Build history of the part. All positions in model axes, mm. A direction names the side the tool comes from. Give positions to 0.01 mm unless a question says otherwise; leave off trailing zeros. Order: outer loops, then holes, each group sorted by start corner. A loop starts at its lowest first (then second) coordinate and runs counter-clockwise, first axis right, second up. Notation, with made-up numbers: (86.5, 33) - (142.5, 33) arc R17 cw to (142.5, 57) - close; hole circle Ø11 at (29, 26.5). An arc over 180 degrees is marked (long way). Use a Markdown table: item, result. Add a question column.
(1) Slice it at A-A (y = 9). Write the cut outline in (x, z), then the cut area to 3 significant figures.
(2) Wall check: line 1 (X direction, y = 3, z = 0); line 2 (X direction, y = 7.75, z = 0); line 3 (Z direction, x = -2, y = 7.25). Give the ranges that are in metal, low to high.
(3) Slice it at B-B (z = 0). Write the cut outline in (x, y) (1 decimal), then the cut area to 3 significant figures.
(4) Flat gauge pins, fed straight in: pin 1 (1 mm diameter, centred on x = -5, y = 6, fed in from +Z); pin 2 (4 mm diameter, centred on y = 9.5, z = -9.5, fed in from -X); pin 3 (6 mm diameter, centred on x = -2, y = 4.5, fed in from -Z); pin 4 (2 mm diameter, centred on x = -7.5, y = 8.5, fed in from -Z). Where does each tip first touch, or does it go through?
(5) Slice it at D-D (x = -7.5). Write the cut outline in (y, z) (3 decimals).
(6) Slice it at C-C (x = 1). Write the cut outline in (y, z) (3 decimals).
(7) Which spindle directions (+Z, -Z, +X, -X, +Y, -Y) get a long thin tool onto all of the face, cutting with end or side? Do faces 4 (the face through (-5.42, 7.58, -9.57)), 5 (the face through (-5.6, 2.19, -7.31)). Say none if no direction does.
(8) Mould opens along X. For faces 1 (the face through (-2, 0, 4)), 2 (the face through (-3.874, 5.322, -0.86)), 3 (the face through (5.58, 7.58, -9.48)) say: +X half, -X half, draft (parallel to the pull), parting line (faces both ways), or undercut.
from build123d import *

# Parameters (mm, degrees)
SKETCH1_R           = 9.2075
SKETCH1_R_2         = 3.96875
BOSS_EXTRUDE1_DEPTH = 4.445
SKETCH2_R           = 3.96875
BOSS_EXTRUDE2_DEPTH = 6.35


with BuildPart() as part:
    # Sketch1 → Boss-Extrude1 (new body)
    with BuildSketch(Plane(origin=(0, 0, 0), x_dir=(1, 0, 0), z_dir=(0, 1, 0))):
        with Locations(Location((0, 0, 0), (0, 0, 270))):  # turned: the seam where the file's is
            Circle(SKETCH1_R)
        with Locations(Location((0, 0, 0), (0, 0, 270))):  # turned: the seam where the file's is
            Circle(SKETCH1_R_2, mode=Mode.SUBTRACT)
    extrude(amount=BOSS_EXTRUDE1_DEPTH)

    # Sketch2 → Boss-Extrude2 (add)
    with BuildSketch(Plane(origin=(0, 4.445, 0), x_dir=(1, 0, 0), z_dir=(0, 1, 0))):
        Polygon((0, 12.7), (-10.998522628, 6.35), (-10.998522628, -6.35), (0, -12.7), (10.998522628, -6.35), (10.998522628, 6.35), align=None)
        with Locations(Location((0, 0, 0), (0, 0, 270))):  # turned: the seam where the file's is
            Circle(SKETCH2_R, mode=Mode.SUBTRACT)
    extrude(amount=BOSS_EXTRUDE2_DEPTH)


solid = part.part
Solution:
| question | item | result |
|---|---|---|
| 1 | outline | (-11, -6.35) - (0, -12.7) - (11, -6.35) - (11, 6.35) - (0, 12.7) - (-11, 6.35) - close; hole circle Ø7.94 at (0, 0) |
| 1 | area | 370 mm2 |
| 2 | line 1 | -9.21 to -3.97, 3.97 to 9.21 |
| 2 | line 2 | -11 to -3.97, 3.97 to 11 |
| 2 | line 3 | -11.55 to -3.43, 3.43 to 11.55 |
| 3 | outline | (-11, 4.4) - (-9.2, 4.4) - (-9.2, 0) - (-4, 0) - (-4, 10.8) - (-11, 10.8) - close; (4, 0) - (9.2, 0) - (9.2, 4.4) - (11, 4.4) - (11, 10.8) - (4, 10.8) - close |
| 3 | area | 136 mm2 |
| 4 | pin 1 | z = 10.1 |
| 4 | pin 2 | x = -9.01 |
| 4 | pin 3 | z = -12.7 |
| 4 | pin 4 | z = -8.95 |
| 5 | outline | (0, -5.341) - (4.445, -5.341) - (4.445, -8.37) - (10.795, -8.37) - (10.795, 8.37) - (4.445, 8.37) - (4.445, 5.341) - (0, 5.341) - close |
| 6 | outline | (0, -9.153) - (4.445, -9.153) - (4.445, -12.123) - (10.795, -12.123) - (10.795, -3.841) - (0, -3.841) - close; (0, 3.841) - (10.795, 3.841) - (10.795, 12.123) - (4.445, 12.123) - (4.445, 9.153) - (0, 9.153) - close |
| 7 | face 4 | -Z, -X, +Y, -Y |
| 7 | face 5 | -Y |
| 8 | face 1 | draft |
| 8 | face 2 | undercut |
| 8 | face 3 | +X half |
